```python
from build123d import *

# Parameters (mm, degrees)
F0_W          = 25
F0_H          = 25
F0_W_2        = 15.5
F0_H_2        = 15.5
F1_DEPTH      = 5
F2_DEPTH      = 25
F2_DEPTH_BACK = 20
F3_SIZE       = 10
F4_SIZE       = 3


with BuildPart() as f1:
    # F0 (on Right) → F1 (new body)
    with BuildSketch(Plane.YZ):
        Polygon((-40.0103315711, 5.9372586757), (-40.0103315711, 30.9372586757), (-15.0103315711, 30.9372586757), (-15.0103315711, 50.9372586757), (-40.0103315711, 50.9372586757), (-90.0103315711, 50.9372586757), (-90.0103315711, 5.9372586757), align=None)
        with BuildLine():
            ThreePointArc((-46.5103315711, 14.4372586757), (-45.4496713993, 13.9979188475), (-45.0103315711, 12.9372586757))
            ThreePointArc((-45.0103315711, 12.9372586757), (-45.4496713993, 11.8765985039), (-46.5103315711, 11.4372586757))
            Line((-46.5103315711, 11.4372586757), (-83.5103315711, 11.4372586757))
            ThreePointArc((-83.5103315711, 11.4372586757), (-85.0103315711, 12.9372586757), (-83.5103315711, 14.4372586757))
            Line((-83.5103315711, 14.4372586757), (-46.5103315711, 14.4372586757))
        make_face(mode=Mode.SUBTRACT)
        with BuildLine():
            ThreePointArc((-62.0103315711, 39.4372586757), (-54.2321569781, 36.2154332687), (-51.0103315711, 28.4372586757))
            ThreePointArc((-51.0103315711, 28.4372586757), (-54.2321569781, 20.6590840826), (-62.0103315711, 17.4372586757))
            Line((-62.0103315711, 17.4372586757), (-68.0103315711, 17.4372586757))
            ThreePointArc((-68.0103315711, 17.4372586757), (-79.0103315711, 28.4372586757), (-68.0103315711, 39.4372586757))
            Line((-68.0103315711, 39.4372586757), (-62.0103315711, 39.4372586757))
        make_face(mode=Mode.SUBTRACT)
        with BuildLine():
            ThreePointArc((-83.5103315711, 42.4372586757), (-85.0103315711, 43.9372586757), (-83.5103315711, 45.4372586757))
            Line((-83.5103315711, 45.4372586757), (-46.5103315711, 45.4372586757))
            ThreePointArc((-46.5103315711, 45.4372586757), (-45.4496713993, 44.9979188475), (-45.0103315711, 43.9372586757))
            ThreePointArc((-45.0103315711, 43.9372586757), (-45.4496713993, 42.8765985039), (-46.5103315711, 42.4372586757))
            Line((-46.5103315711, 42.4372586757), (-83.5103315711, 42.4372586757))
        make_face(mode=Mode.SUBTRACT)
        with Locations((-27.5103315711, 18.4372586757)):
            Rectangle(F0_W, F0_H)
        with Locations((-27.5103315711, 18.4372586757)):
            Rectangle(F0_W_2, F0_H_2, mode=Mode.SUBTRACT)
    extrude(amount=F1_DEPTH)

    # F0 (on Right) → F2 (join, two sides)
    with BuildSketch(Plane.YZ) as f2_sk:
        with Locations((-27.5103315711, 18.4372586757)):
            Rectangle(F0_W, F0_H)
        with Locations((-27.5103315711, 18.4372586757)):
            Rectangle(F0_W_2, F0_H_2, mode=Mode.SUBTRACT)
    extrude(amount=F2_DEPTH)
    extrude(f2_sk.sketch, amount=-F2_DEPTH_BACK)

    # F3
    f3_edges = [f1.edges().sort_by_distance(p)[0] for p in [
        (5, -27.510332, 30.937259),
        (0, -27.510332, 30.937259),
    ]]
    chamfer(f3_edges, length=F3_SIZE)

    # F4
    f4_edges = [f1.edges().sort_by_distance(p)[0] for p in [
        (2.5, -15.010332, 5.937259),
        (-15, -15.010332, 30.937259),
        (20, -15.010332, 30.937259),
    ]]
    chamfer(f4_edges, length=F4_SIZE)


solid = f1.part
```
Part model, mm, in its own coordinate system. A direction names the side the tool comes from. Give positions to 0.01 mm unless a question says otherwise; leave off trailing zeros. Write each loop counter-clockwise with the first axis right and the second up, starting at its lowest first coordinate (ties: lowest second). Pieces come first, ordered by that corner, then holes. Notation, with made-up numbers: (69, -34) -> (97, -34) arc R21 cw to (97, -25) -> close; hole circle Ø8 at (33, 75.5). An arc over 180 degrees is marked (long way). Put each result on its own line as item: value. Start each with the question number.
Item 1: Cut at A-A (y = -24). List the corners of the cut face in (x, z), then the cut area to 4 significant figures.
Item 2: Cut at C-C (z = 16.5). List the corners of the cut face in (x, y).
Item 3: Pin check, flat tips, straight feed: pin 1 Ø2 at (y, z) = (-66.5, 13) entering from +X; pin 2 Ø8 at (x, z) = (-15.5, 32) entering from +Y; pin 3 Ø5 at (x, z) = (-13.5, 16.5) entering from -Y; pin 4 Ø5 at (x, y) = (-16.5, -34) entering from +Z. Stop position of each tip, or through.
Item 4: Pull direction Z, two halves, no side cores. Call faces 4 (the face through (2, -65, 14.437)), 5 (the face through (2, -52, 50.937)), 6 (the face through (0, -53, 39)): pulls with the +Z half, pulls with the -Z half, needs draft (parallel to the pull), parting line crosses it, or undercut.
Item 5: Which spindle directions (+Z, -Z, +X, -X, +Y, -Y) get a long thin tool onto all of the face, cutting with end or side? Do faces 1 (the face through (20, -29, 30.937)), 2 (the face through (2.46, -85.01, 43.9)), 3 (the face through (21.041, -16.489, 29.416)). Say none if no direction does.
Item 6: Cut at D-D (y = -76.5). List the corners of the cut face in (x, z), then the cut area to 3 significant figures.
Item 7: Wall check: L1, parallel to Z at x = 1, y = -63; L2, parallel to Z at x = 15.5, y = -32; L3, parallel to Y at x = -9, z = 22.5. Give the ranges that are in metal, low to high. Write a range as [from, to].
Item 8: Cut at B-B (x = 2). List the corners of the cut face in (y, z), then the cut area to 3 significant figures.
Answer list:
1. outline: (-20, 5.94) -> (25, 5.94) -> (25, 10.69) -> (-20, 10.69) -> close; (-20, 26.19) -> (25, 26.19) -> (25, 30.94) -> (15, 30.94) -> (5, 40.94) -> (5, 50.94) -> (0, 50.94) -> (0, 40.94) -> (-10, 30.94) -> (-20, 30.94) -> close
1. area: 627.5 mm2
2. outline: (-20, -40.01) -> (0, -40.01) -> (0, -90.01) -> (5, -90.01) -> (5, -40.01) -> (25, -40.01) -> (25, -35.26) -> (-20, -35.26) -> close; (-20, -19.76) -> (25, -19.76) -> (25, -15.01) -> (-20, -15.01) -> close
3. pin 1: passes through
3. pin 2: stops at y = -15.07
3. pin 3: stops at y = -40.01
3. pin 4: stops at z = 30.94
4. face 4: undercut
4. face 5: pulls with the +Z half
4. face 6: needs draft
5. face 1: +Z, +X, +Y, -Y
5. face 2: +X, -X
5. face 3: +Z, +X, +Y
6. outline: (0, 5.94) -> (5, 5.94) -> (5, 11.44) -> (0, 11.44) -> close; (0, 14.44) -> (5, 14.44) -> (5, 21.44) -> (0, 21.44) -> close; (0, 35.43) -> (5, 35.43) -> (5, 42.44) -> (0, 42.44) -> close; (0, 45.44) -> (5, 45.44) -> (5, 50.94) -> (0, 50.94) -> close
6. area: 125 mm2
7. L1: z = [5.94, 11.44], [14.44, 17.44], [39.44, 42.44], [45.44, 50.94]
7. L2: z = [5.94, 10.69], [26.19, 30.94]
7. L3: y = [-40.01, -35.26], [-19.76, -15.01]
8. outline: (-90.01, 5.94) -> (-18.01, 5.94) -> (-15.01, 8.94) -> (-15.01, 50.94) -> (-90.01, 50.94) -> close; hole (-83.51, 11.44) -> (-46.51, 11.44) arc R1.5 ccw to (-46.51, 14.44) -> (-83.51, 14.44) arc R1.5 ccw to start; hole (-83.51, 42.44) -> (-46.51, 42.44) arc R1.5 ccw to (-46.51, 45.44) -> (-83.51, 45.44) arc R1.5 ccw to start; hole (-68.01, 17.44) -> (-62.01, 17.44) arc R11 ccw to (-62.01, 39.44) -> (-68.01, 39.44) arc R11 ccw to start; hole (-35.26, 10.69) -> (-19.76, 10.69) -> (-19.76, 26.19) -> (-35.26, 26.19) -> close
8. area: 2,380 mm2
